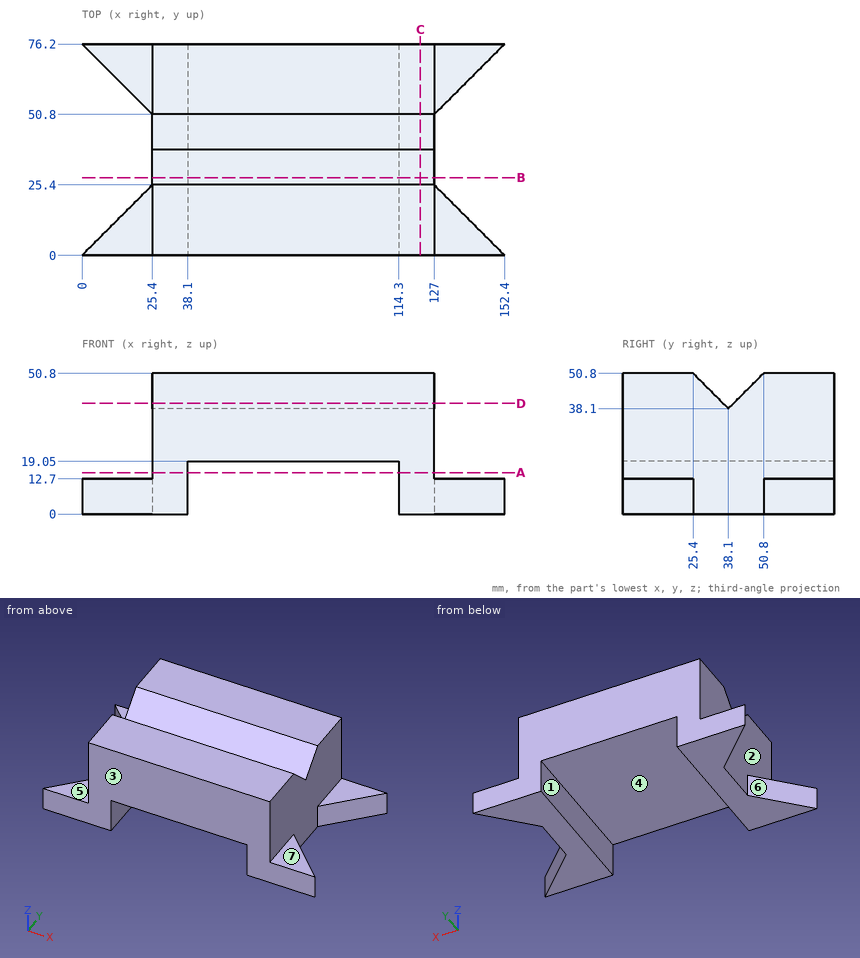
Design review of the part shown in the three views and the two pictorial views. Dimensions are in mm from the part's minimum x, y and z. A direction names the side the tool comes from. Round coordinates to 2 decimals unless told otherwise and drop trailing zeros. Loops run counter-clockwise (first coordinate to the right, second up) from the corner with the lowest first, then second, coordinate; pieces in that order, holes last. Notation, with made-up numbers: (54, 74.5) -> (112, 74.5) arc R27 cw to (112, 98.5) -> close; hole circle Ø6 at (11, -18.75). An arc over 180 degrees is marked (long way). Use one line per item in the form item = value. Start each with the question number.
Q1. Draft analysis for pull direction X (two halves, no side actions). For the marked faces 1, 2, 3 and 4, state which applies: +X half, -X half, draft (parallel to the pull), parting line (faces both ways), or undercut.
Q2. We need section B-B on y = 28. Give the boundary of the cut face in (x, z), then the cut area to 3 significant figures.
Q3. Wall thickness on line 1 along X through (y, z) = (57, 14); line 2 along Z through (x, y) = (75.5, 60.5); line 3 along Z through (x, y) = (16.5, 70): over which ranges is each line inside the solid? List them lowest first. Write a range as [from, to].
Q4. We need section A-A on z = 15. Give the boundary of the cut face in (x, y).
Q5. We need section D-D on z = 40. Give the boundary of the cut face in (x, y).
Q6. Machinability: for the marked faces 5, 6 and 7, which of the approach directions +Z, -Z, +X, -X, +Y, -Y give a long, thin tool a straight path to every point of the face, cutting with its end or side? Answer none if there is none.
Q7. For pin 1 Ø12.5 at (x, y) = (143.5, 68.5) entering from +Z; pin 2 Ø9.5 at (y, z) = (47, 8.5) entering from -X; pin 3 Ø5.5 at (y, z) = (47.5, 13) entering from +X; pin 4 Ø20.5 at (x, y) = (15.5, 59.5) entering from +Z, all flat-tipped, find the tip position at first contact; note any pin that passes through.
Q8. We need section C-C on x = 122. Give the boundary of the cut face in (y, z), then the cut area to 3 significant figures.
Calculated:
q1.face_1 = undercut
q1.face_2 = -X half
q1.face_3 = draft
q1.face_4 = undercut
q2.outline = (25.4, 0) -> (38.1, 0) -> (38.1, 19.05) -> (114.3, 19.05) -> (114.3, 0) -> (127, 0) -> (127, 48.2) -> (25.4, 48.2) -> close
q2.area = 3,450 mm²
q3.line_1 = [25.4, 38.1], [114.3, 127]
q3.line_2 = [19.05, 50.8]
q3.line_3 = [0, 12.7]
q4.outline = (25.4, 0) -> (38.1, 0) -> (38.1, 76.2) -> (25.4, 76.2) -> close; (114.3, 0) -> (127, 0) -> (127, 76.2) -> (114.3, 76.2) -> close
q5.outline = (25.4, 0) -> (127, 0) -> (127, 36.2) -> (25.4, 36.2) -> close; (25.4, 40) -> (127, 40) -> (127, 76.2) -> (25.4, 76.2) -> close
q6.face_5 = +Z, -X, +Y, -Y
q6.face_6 = +Z, -Z, -X
q6.face_7 = +Z, +X, +Y, -Y
q7.pin_1 = 12.7
q7.pin_2 = 24.45
q7.pin_3 = 127
q7.pin_4 = 50.8
q8.outline = (0, 0) -> (76.2, 0) -> (76.2, 50.8) -> (50.8, 50.8) -> (38.1, 38.1) -> (25.4, 50.8) -> (0, 50.8) -> close
q8.area = 3,710 mm²
